The drawing under review shows one solid part. Ordinate dimensions are in mm from its lowest x, y, z. A direction names the side the tool comes from. Coordinates: 2 decimals unless noted, no trailing zeros. Write each loop counter-clockwise with the first axis right and the second up, starting at its lowest first coordinate (ties: lowest second). Pieces come first, ordered by that corner, then holes.
Q1. Clearance check with flat-ended pins moving along their axes: pin 1 Ø2 at (y, z) = (3, 20.5) entering from -X; pin 2 Ø4.5 at (x, z) = (11, 20) entering from +Y; pin 3 Ø7 at (x, y) = (171, 10) entering from -Z; pin 4 Ø12 at (x, z) = (86, 19.5) entering from +Y. State where each tip first meets the part, or that it passes through.
Q2. The part is to be moulded in two halves that separate along Z. For the marked faces 1, 2 and 3, say which applies: +Z half, -Z half, draft (parallel to the pull), parting line (faces both ways), or undercut.
Q3. Add section B-B, the plane x = 171. Give the boundary of the cut face in (y, z), plus the area to 3 significant figures.
Q4. Machinability: for the marked faces 4 and 5, which of the approach directions +Z, -Z, +X, -X, +Y, -Y give a long, thin tool a straight path to every point of the face, cutting with its end or side? Answer none if there is none.
Q5. Add section A-A, the plane z = 30.5. Give the boundary of the cut face in (x, y), plus the area to 3 significant figures.
Q6. Add section C-C, the plane y = 10. Give the boundary of the cut face in (x, z).
Q7. Add section D-D, the plane x = 117. Give the boundary of the cut face in (y, z).
Q8. To check wall thickness, follow probe 1 along X at (y, z) = (2.5, 11); probe 2 along Y at (x, z) = (171, 39); probe 3 along X at (y, z) = (4.5, 2.5). State the ranges of each line that lie inside material, in increasing order.
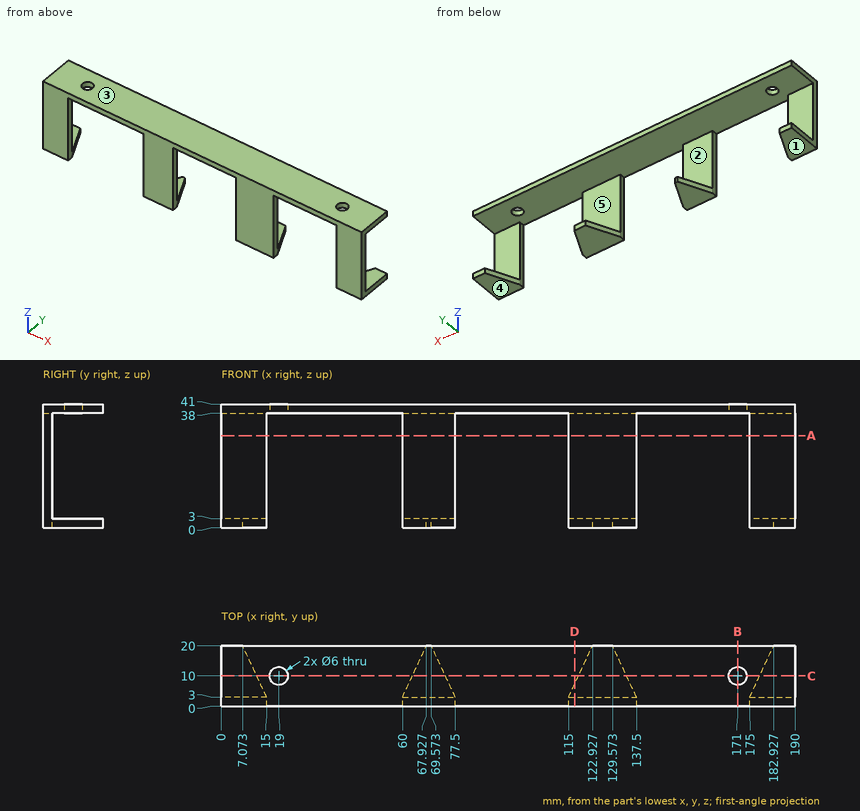
Here are the results:
1. pin 1: stops at x = 0
1. pin 2: stops at y = 3
1. pin 3: stops at z = 38
1. pin 4: passes through
2. face 1: -Z half
2. face 2: undercut
2. face 3: +Z half
3. outline: (0, 38) - (7, 38) - (7, 41) - (0, 41) - close; (13, 38) - (20, 38) - (20, 41) - (13, 41) - close
3. area: 42.0 mm2
4. face 4: -Z, +X, -X, +Y, -Y
4. face 5: +X, -X, +Y
5. outline: (0, 0) - (15, 0) - (15, 3) - (0, 3) - close; (60, 0) - (77.5, 0) - (77.5, 3) - (60, 3) - close; (115, 0) - (137.5, 0) - (137.5, 3) - (115, 3) - close; (175, 0) - (190, 0) - (190, 3) - (175, 3) - close
5. area: 210 mm2
6. outline: (0, 0) - (11.74, 0) - (11.74, 3) - (0, 3) - close; (0, 38) - (16, 38) - (16, 41) - (0, 41) - close; (22, 38) - (168, 38) - (168, 41) - (22, 41) - close; (63.26, 0) - (74.24, 0) - (74.24, 3) - (63.26, 3) - close; (118.26, 0) - (134.24, 0) - (134.24, 3) - (118.26, 3) - close; (174, 38) - (190, 38) - (190, 41) - (174, 41) - close; (178.26, 0) - (190, 0) - (190, 3) - (178.26, 3) - close
7. outline: (0, 0) - (7.29, 0) - (7.29, 3) - (3, 3) - (3, 38) - (20, 38) - (20, 41) - (0, 41) - close
8. probe 1: x = 0 to 15, 60 to 77.5, 115 to 137.5, 175 to 190
8. probe 2: y = 0 to 7, 13 to 20
8. probe 3: x = 0 to 14.3, 60.7 to 76.8, 115.7 to 136.8, 175.7 to 190
